The figure shows three views and two pictorial views of one solid part (mm, origin at its lowest corner). Answer the questions. Give positions to 0.01 mm unless a question says otherwise; leave off trailing zeros. Order: outer loops, then holes, each group sorted by start corner. A loop starts at its lowest first (then second) coordinate and runs counter-clockwise, first axis right, second up. Notation, with made-up numbers: (-8, 63) - (22, 63) arc R11 cw to (22, 76) - close; hole circle Ø1 at (45.25, -11.75). An arc over 180 degrees is marked (long way). Answer as a JSON object with one key per item and string values. Group by question number.
Q1. A cutting plane is placed at C-C, the plane y = 300. Give the vertices of the cut face in (x, z), and give its area (4 significant figures).
Q2. A cutting plane is placed at A-A, the plane z = 20. Give the vertices of the cut face in (x, y).
Q3. Given pin 1 (1 mm diameter, centred on x = 2.5, y = 140, fed in from +Z), flat-ended and moving along its own axis, determine where the tip first touches the part or whether it passes through.
Q4. Consider line 1 (Y direction, x = 2.9, z = 60); line 2 (Z direction, x = 1.4, y = 300); line 3 (Z direction, x = 3.1, y = 270). Determine where each line is inside the solid, lowest interval first.
Q5. A cutting plane is placed at D-D, the plane y = 240. Give the vertices of the cut face in (x, z).
Q6. A cutting plane is placed at B-B, the plane x = 1.2. Count the separate pieces of the cut face and the enclosed holes in it, and give its area (3 significant figures).
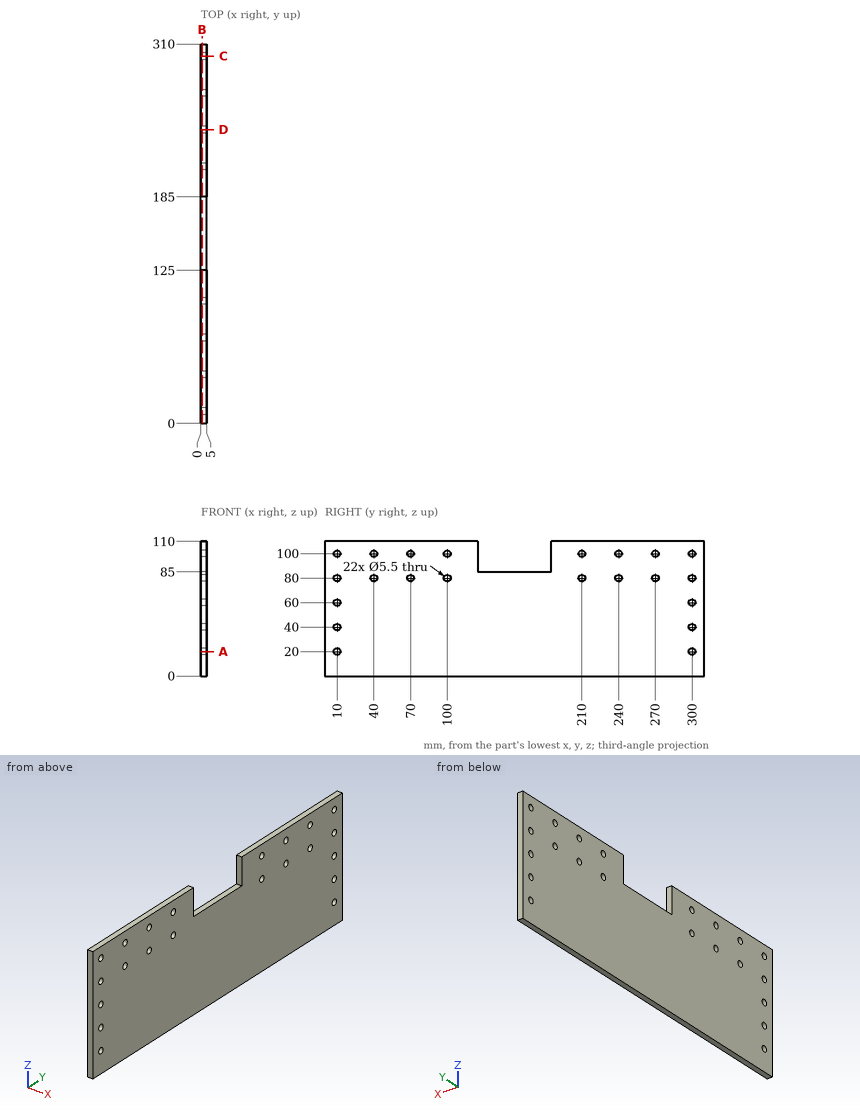
Reply:
{
 "1": {"outline": "(0, 0) - (5, 0) - (5, 17.25) - (0, 17.25) - close; (0, 22.75) - (5, 22.75) - (5, 37.25) - (0, 37.25) - close; (0, 42.75) - (5, 42.75) - (5, 57.25) - (0, 57.25) - close; (0, 62.75) - (5, 62.75) - (5, 77.25) - (0, 77.25) - close; (0, 82.75) - (5, 82.75) - (5, 97.25) - (0, 97.25) - close; (0, 102.75) - (5, 102.75) - (5, 110) - (0, 110) - close", "area": "412.5 mm^2"},
 "2": {"outline": "(0, 0) - (5, 0) - (5, 7.25) - (0, 7.25) - close; (0, 12.75) - (5, 12.75) - (5, 297.25) - (0, 297.25) - close; (0, 302.75) - (5, 302.75) - (5, 310) - (0, 310) - close"},
 "3": {"pin 1": "stops at z = 85"},
 "4": {"line 1": "y = 0 to 7.25, 12.75 to 297.25, 302.75 to 310", "line 2": "z = 0 to 17.25, 22.75 to 37.25, 42.75 to 57.25, 62.75 to 77.25, 82.75 to 97.25, 102.75 to 110", "line 3": "z = 0 to 77.25, 82.75 to 97.25, 102.75 to 110"},
 "5": {"outline": "(0, 0) - (5, 0) - (5, 77.25) - (0, 77.25) - close; (0, 82.75) - (5, 82.75) - (5, 97.25) - (0, 97.25) - close; (0, 102.75) - (5, 102.75) - (5, 110) - (0, 110) - close"},
 "6": {"separate pieces": "1", "enclosed holes": "22", "area": "32,100 mm^2"}
}
